Can you work these out from the drawing? Everything is in mm from the part's minimum corner. Coordinates: 2 decimals unless noted, no trailing zeros. Write each loop counter-clockwise with the first axis right and the second up, starting at its lowest first coordinate (ties: lowest second). Pieces come first, ordered by that corner, then holes. Notation, with made-up numbers: M 13.5,9 L 51.5,9 A11 cw 51.5,30 Z; hole C -10.5,-8.5 d4. An arc over 180 degrees is marked long. Write each question's results on one line, items separated by ' | '. Start each with the question number.
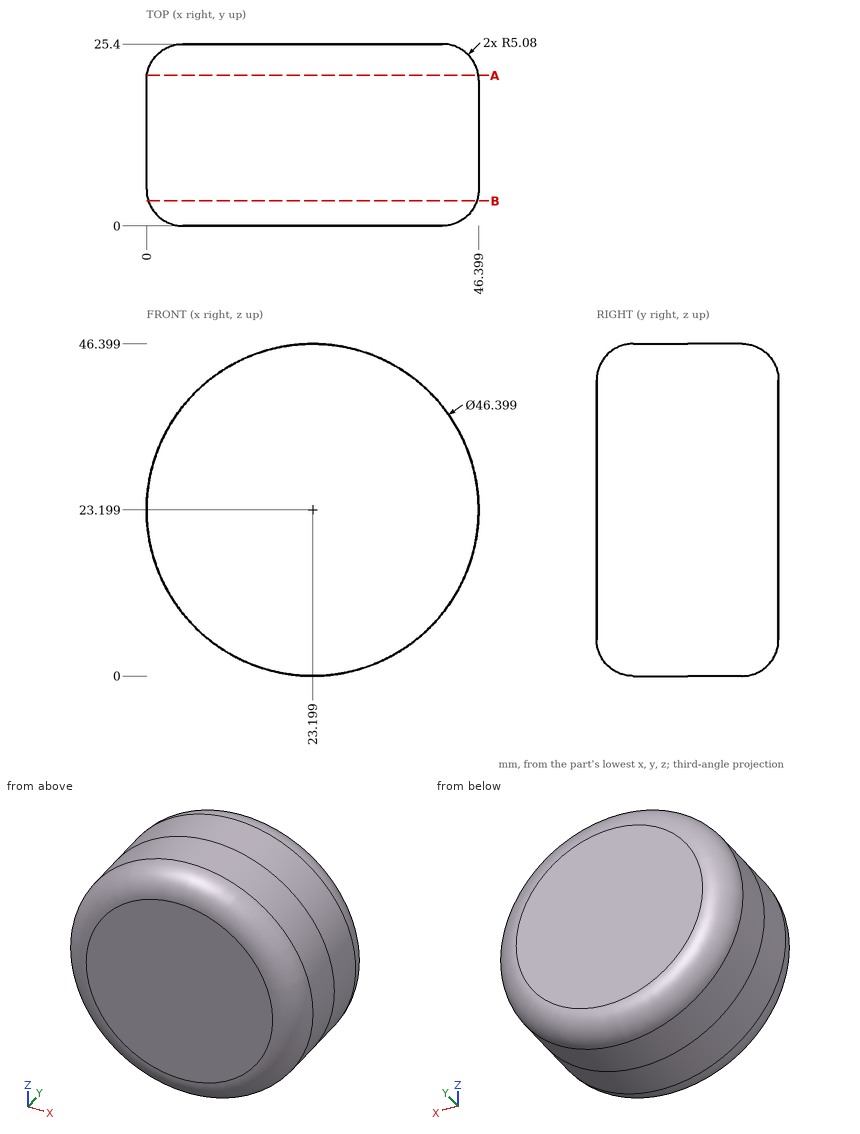
1) For pin 1 Ø6 at (y, z) = (17.5, 18.5) entering from +X; pin 2 Ø1 at (x, y) = (22.5, 8.5) entering from +Z; pin 3 Ø8 at (y, z) = (16.5, 36.5) entering from -X, each with a flat end and sliding along its axis, tell me the tip position at first contact or that it passes through.
2) I want a section at A-A, the plane y = 21. Write out the boundary of the cut face in (x, z) (1 decimal).
3) Please list where these lines run through material, in increasing order: line 1 (Y direction, x = 31.5, z = 7); line 2 (Z direction, x = 35.5, y = 15.75); line 3 (Y direction, x = 18, z = 4). Write a range as [from, to].
4) I want a section at B-B, the plane y = 3.5. Write out the boundary of the cut face in (x, z) (1 decimal), then the cut area to 3 significant figures.
Output:
1) pin 1: stops at x = 46.34 | pin 2: stops at z = 46.4 | pin 3: stops at x = 1.95
2) outline: C 23.2,23.2 d46.3
3) line 1: y = [0, 25.4] | line 2: z = [3.53, 42.87] | line 3: y = [0.32, 25.08]
4) outline: C 23.2,23.2 d45.9 | area: 1,650 mm2
